```python
from build123d import *

# Parameters (mm, degrees)
SKETCH1_W           = 158.75
SKETCH1_H           = 25.4
BOSS_EXTRUDE1_DEPTH = 3.175
SKETCH2_R           = 1.5875
SKETCH2_W           = 3.175
SKETCH2_H           = 12.7
CUT_EXTRUDE1_DEPTH  = 4.175


with BuildPart() as part:
    # Sketch1 → Boss-Extrude1 (new body)
    with BuildSketch(Plane(origin=(0, 0, 0), x_dir=(0, 0, -1), z_dir=(1, 0, 0))):
        with Locations((79.375, 12.7)):
            Rectangle(SKETCH1_W, SKETCH1_H)
    extrude(amount=BOSS_EXTRUDE1_DEPTH)

    # Sketch2 → Cut-Extrude1 (cut, through all)
    with BuildSketch(Plane.ZY):
        with Locations((-97.917, 12.7)):
            Circle(SKETCH2_R)
        with Locations((-60.833, 12.7)):
            Circle(SKETCH2_R)
        with Locations((-1.5875, 6.35)):
            Rectangle(SKETCH2_W, SKETCH2_H)
        with Locations((-157.1625, 6.35)):
            Rectangle(SKETCH2_W, SKETCH2_H)
    extrude(amount=-CUT_EXTRUDE1_DEPTH, mode=Mode.SUBTRACT)


solid = part.part
```
Part model, mm, in its own coordinate system. A direction names the side the tool comes from. Round coordinates to 2 decimals unless told otherwise and drop trailing zeros. Write each loop counter-clockwise with the first axis right and the second up, starting at its lowest first coordinate (ties: lowest second). Pieces come first, ordered by that corner, then holes.
Item 1: Probe L1, parallel to Z at x = 2.45, y = 5 (3 decimals); L2, parallel to Y at x = 2.55, z = -97; L3, parallel to Z at x = 2, y = 11.5 (3 decimals). List the from-to ranges inside material, lowest first.
Results:
L1: z = -155.575 to -3.175
L2: y = 0 to 11.4, 14 to 25.4
L3: z = -155.575 to -98.956, -96.878 to -61.872, -59.794 to -3.175
Item 2: Cut at B-B, the plane y = 6.5. Give the cut face in (x, z) (3 decimals).
Results:
outline: (0, -155.575) - (3.175, -155.575) - (3.175, -3.175) - (0, -3.175) - close
Item 3: Cut at A-A, the plane x = 1.4. Count the separate pieces of the cut face and the enclosed holes in it, plus the area to 3 significant figures.
Results:
separate pieces: 1
enclosed holes: 2
area: 3,940 mm2
Item 4: Two-plate mould, pull along Y, no slides. Class faces 4 (the flat face through (2, 12.7, -157)), 5 (the flat face through (0, 13, -78)), 6 (the cylindrical face through (1.57, 12.09, -96.45)): +Y half, -Y half, draft (parallel to the pull), parting line (faces both ways), or undercut.
Results:
face 4: -Y half
face 5: draft
face 6: undercut
Item 5: Drop flat-ended pins along their axis: pin 1 Ø1 at (x, y) = (1, 4.5) entering from -Z (3 decimals); pin 2 Ø2.5 at (y, z) = (12.7, -60.833) entering from +X; pin 3 Ø4 at (y, z) = (12.7, -97.917) entering from +X (3 decimals); pin 4 Ø1.6 at (x, z) = (2, -1) entering from -Y. Give the stop position or say it passes through.
Results:
pin 1: stops at z = -155.575
pin 2: passes through
pin 3: stops at x = 3.175
pin 4: stops at y = 12.7
Item 6: Which spindle directions (+Z, -Z, +X, -X, +Y, -Y) get a long thin tool onto all of the face, cutting with end or side? Do faces 1 (the flat face through (2, 6, -155.575)), 2 (the flat face through (2, 6, -3.175)), 3 (the flat face through (3.175, 13, -78)). Say none if no direction does.
Results:
face 1: -Z, +X, -X, -Y
face 2: +Z, +X, -X, -Y
face 3: +Z, -Z, +X, +Y, -Y
